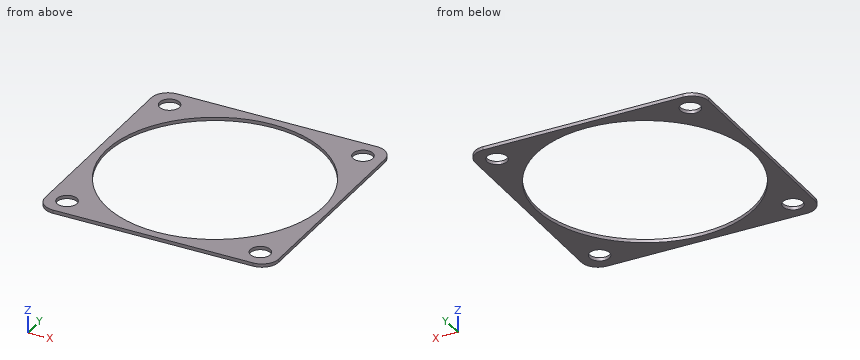
Autodesk Fusion 360 part; units mm, degrees
sketch "Sketch1" plane through (0, 0, 0) normal (0, 0, 1) x (1, 0, 0)
  line L0 (30, -35) -> (-30, -35)
  line L1 (-35, -30) -> (-35, 30)
  line L2 (-30, 35) -> (30, 35)
  line L3 (35, 30) -> (35, -30)
  line L4 (35, -35) -> (-35, 35) construction
  line L5 (-35, -35) -> (35, 35) construction
  circle A0 centre (0, 0) radius 32.5
  circle A1 centre (-28.9896, 28.9896) radius 3
  arc A2 (-30, 35) -> (-35, 30) centre (-30, 30) ccw
  arc A3 (35, 30) -> (30, 35) centre (30, 30) ccw
  arc A4 (30, -35) -> (35, -30) centre (30, -30) ccw
  arc A5 (-35, -30) -> (-30, -35) centre (-30, -30) ccw
  line L6 (0, 35) -> (0, -35) construction
  line L7 (-35, 0) -> (35, 0) construction
  circle A6 centre (28.9896, 28.9896) radius 3
  circle A7 centre (-28.9896, -28.9896) radius 3
  circle A8 centre (28.9896, -28.9896) radius 3
  dimension "d1" = 70
  dimension "d2" = 70
  dimension "d3" = 65
  dimension "d4" = 6
  dimension "d5" = 8.5
  dimension "d6" = 5
  dimension "d7" = 5
  dimension "d8" = 5
  dimension "d9" = 5
extrude "Extrude1" add sketch "Sketch1" along normal blind 1
Here's how the part is built. I have some questions about the finished solid (model axes, mm). Give positions to 0.01 mm unless a question says otherwise; leave off trailing zeros. Loops run counter-clockwise (first coordinate to the right, second up) from the corner with the lowest first, then second, coordinate; pieces in that order, holes last. Notation, with made-up numbers: M 4,71 L 55,71 A19 cw 55,97 Z; hole C -7.75,66.25 d1. An arc over 180 degrees is marked long. Return JSON: item names as keys, results as strings.
Item 1: Please list where these lines run through material, in increasing order: line 1 (Y direction, x = 1, z = 0.1); line 2 (X direction, y = 29, z = 0.6); line 3 (Y direction, x = -19, z = 0.4).
A:
{"line 1": "y = -35 to -32.48, 32.48 to 35", "line 2": "x = -35 to -31.99, -25.99 to -14.67, 14.67 to 25.99, 31.99 to 35", "line 3": "y = -35 to -26.37, 26.37 to 35"}
Item 2: I'm going to push a flat-ended pin straight in: pin 1 Ø3.5 at (x, y) = (-28.99, 28.99) entering from -Z. Where does the tip first touch, or does it pass through?
A:
{"pin 1": "passes through"}
Item 3: Imagine slicing it at A-A on y = 0. List the corners of the cut face in (x, z) for me.
A:
{"outline": "M -35,0 L -32.5,0 L -32.5,1 L -35,1 Z; M 32.5,0 L 35,0 L 35,1 L 32.5,1 Z"}
Item 4: Imagine slicing it at C-C on z = 0.2. List the corners of the cut face in (x, y) for me, then the cut area to 3 significant figures.
A:
{"outline": "M -35,-30 A5 ccw -30,-35 L 30,-35 A5 ccw 35,-30 L 35,30 A5 ccw 30,35 L -30,35 A5 ccw -35,30 Z; hole C 0,0 d65; hole C -28.99,-28.99 d6; hole C -28.99,28.99 d6; hole C 28.99,-28.99 d6; hole C 28.99,28.99 d6", "area": "1,450 mm^2"}
